Part model, mm, in its own coordinate system. A direction names the side the tool comes from. Give positions to 0.01 mm unless a question says otherwise; leave off trailing zeros. Order: outer loops, then holes, each group sorted by start corner. A loop starts at its lowest first (then second) coordinate and runs counter-clockwise, first axis right, second up. Notation, with made-up numbers: M -39,49 L -18,49 A10 ccw -18,53 Z; hole C 32.25,61.25 d5. An arc over 180 degrees is marked long. Return JSON: item names as keys, results as strings.
from build123d import *

# Parameters (mm, degrees)
F1_DEPTH = 38.1
F2_DEPTH = 38.1


with BuildPart() as f1:
    # F0 (on Front) → F1 (new body)
    with BuildSketch(Plane.XZ):
        Polygon((-101.6, 50.8), (-101.6, 0), (50.8, 0), (50.8, 50.8), (25.4, 50.8), (25.4, 25.4), (0, 25.4), (0, 50.8), align=None)
    extrude(amount=-F1_DEPTH)

    # F1_face (on face) → F2 (join)
    with BuildSketch(Plane(origin=(-28.863636, 0, 24.245455), x_dir=(1, 0, 0), z_dir=(0, -1, 0))):
        Polygon((-72.736364, -24.245455), (79.663636, -24.245455), (79.663636, 26.554545), (54.263636, 26.554545), (54.263636, 1.154545), (28.863636, 1.154545), (28.863636, 26.554545), (-72.736364, 26.554545), align=None)
    extrude(amount=F2_DEPTH)


solid = f1.part
Q1. Band-saw the part on C-C (x = 8.5). Give the cut face in (y, z), then the cut area to 3 significant figures.
Established:
{"outline": "M -38.1,0 L 38.1,0 L 38.1,25.4 L -38.1,25.4 Z", "area": "1,940 mm²"}
Q2. Two-plate mould, pull along X, no slides. Class faces 1 (the flat face through (-101.6, 1, 26)), 2 (the flat face through (-50, 1, 50.8)), 3 (the flat face through (25.4, 1, 38)): +X half, -X half, draft (parallel to the pull), parting line (faces both ways), or undercut.
Established:
{"face 1": "-X half", "face 2": "draft", "face 3": "undercut"}
Q3. Band-saw the part on B-B (y = 22). Give the cut face in (x, z), then the cut area to 3 significant figures.
Established:
{"outline": "M -101.6,0 L 50.8,0 L 50.8,50.8 L 25.4,50.8 L 25.4,25.4 L 0,25.4 L 0,50.8 L -101.6,50.8 Z", "area": "7,100 mm²"}
Q4. Probe line 1 along X through (y, z) = (-18.5, 32); line 2 along Z through (x, y) = (17, -9.5). List the from-to ranges inside material, lowest first.
Established:
{"line 1": "x = -101.6 to 0, 25.4 to 50.8", "line 2": "z = 0 to 25.4"}
Q5. 3-axis set-ups, long thin cutter, end or side, ignore diameter. For faces 4 (the flat face through (-26, 38.1, 26)), 5 (the flat face through (0, 1, 38)): which of +Z, -Z, +X, -X, +Y, -Y reach the whole face in a straight line?
Established:
{"face 4": "+Z, -Z, +X, -X, +Y", "face 5": "+Z, +Y, -Y"}
Q6. Band-saw the part on A-A (z = 33.5). Give the cut face in (x, y), then the cut area to 3 significant figures.
Established:
{"outline": "M -101.6,-38.1 L 0,-38.1 L 0,38.1 L -101.6,38.1 Z; M 25.4,-38.1 L 50.8,-38.1 L 50.8,38.1 L 25.4,38.1 Z", "area": "9,680 mm²"}
